Geometry: see drawing. Coordinates: mm, zero at the bounding-box minimum. Round coordinates to 2 decimals unless told otherwise and drop trailing zeros. Loops run counter-clockwise (first coordinate to the right, second up) from the corner with the lowest first, then second, coordinate; pieces in that order, holes last.
(1) Cut plane B-B, the plane y = 23. Output: boundary loops of the cut face in (x, z).
(2) Line query: line 1 (X direction, y = 23.5, z = 0.25); line 2 (X direction, y = 5.5, z = 0.15); line 3 (X direction, y = 30, z = 0.15). Output: solid intervals per line, ascending.
(3) Cut plane A-A, the plane x = 83. Output: boundary loops of the cut face in (y, z) (3 decimals).
(4) First-contact query: pin 1 Ø1.1 at (x, z) = (95.5, 1.5) entering from -Y; pin 2 Ø2.5 at (x, y) = (57.023, 69.723) entering from +Z; pin 3 Ø1.1 at (y, z) = (24, 0.5) entering from +X. Flat tips, straight axial feed; report the tip coordinate or a pass-through.
(5) Cut plane D-D, the plane z = 1. Give the number of separate pieces and of enclosed holes in the cut face, and give its area (3 significant figures).
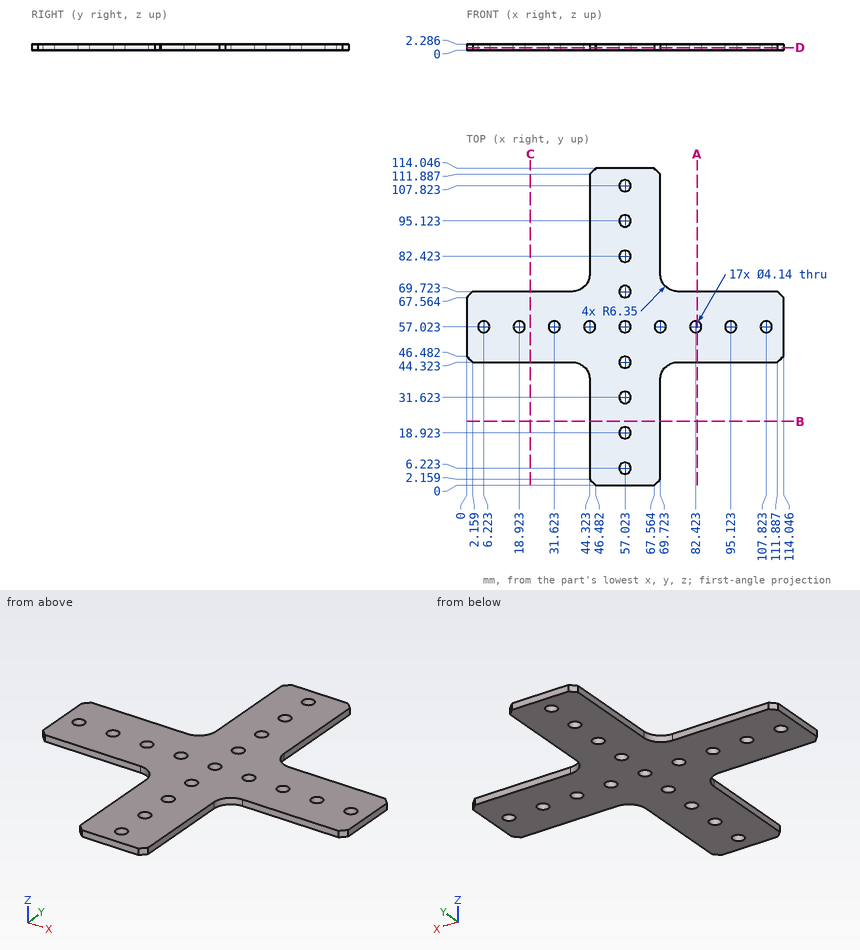
Reported:
1. outline: (44.32, 0) - (69.72, 0) - (69.72, 2.29) - (44.32, 2.29) - close
2. line 1: x = 44.32 to 69.72
2. line 2: x = 44.32 to 55.08, 58.96 to 69.72
2. line 3: x = 44.32 to 55.74, 58.31 to 69.72
3. outline: (44.323, 0) - (55.035, 0) - (55.035, 2.286) - (44.323, 2.286) - close; (59.011, 0) - (69.723, 0) - (69.723, 2.286) - (59.011, 2.286) - close
4. pin 1: stops at y = 44.32
4. pin 2: passes through
4. pin 3: stops at x = 69.72
5. separate pieces: 1
5. enclosed holes: 17
5. area: 4,940 mm2
